```python
from build123d import *

# Parameters (mm, degrees)
SKETCH_2_R               = 2.1
SKETCH_2_R_2             = 4.1
EXTRUDE_2_DEPTH          = 3
EXTRUDE_3_DEPTH          = 15
SKETCH_4_R               = 4.1
SKETCH_4_R_2             = 2.1
EXTRUDE_4_DEPTH          = 10
EXTRUDE_START            = -13
EXTRUDE_5_DEPTH          = 13
SKETCH_7_R               = 1.3
CUT_EXTRUDE_1_DEPTH      = 13
CUT_EXTRUDE_2_DEPTH      = 174.68818701
CUT_EXTRUDE_2_DEPTH_BACK = 174.68818701
SKETCH_8_W               = 110
SKETCH_8_H               = 2.6
SKETCH_8_H_2             = 2.5
CUT_EXTRUDE_3_DEPTH      = 172.969913078
CUT_EXTRUDE_3_DEPTH_BACK = 172.969913078
EXTRUDE_6_DEPTH          = 10
SKETCH_11_R              = 2
CUT_EXTRUDE_4_DEPTH      = 10
SKETCH_13_R              = 2.05
CUT_EXTRUDE_5_DEPTH      = 10
SKETCH_14_R              = 4.1
EXTRUDE_7_DEPTH          = 3
CUT_EXTRUDE_6_DEPTH      = 3


# Read off the part's stored shape, not the designer's step: 凸台-拉伸3, 凸台-拉伸5
with BuildPart() as part:
    # 草图2 → 凸台-拉伸2 (new body)
    with BuildSketch(Plane(origin=(0, 0, 0), x_dir=(1, 0, 0), z_dir=(0, 1, 0))):
        with BuildLine():
            Line((80.099742919, 115.241133642), (-11.337123868, 9.698254241))
            ThreePointArc((-11.337123868, 9.698254241), (-10.606601718, -10.730242528), (9.821895051, -11.460764678))
            Line((9.821895051, -11.460764678), (115.364774452, 79.976102109))
            ThreePointArc((115.364774452, 79.976102109), (115.409508589, 80.014950331), (115.454150533, 80.053904459))
            Line((115.454150533, 80.053904459), (113.400395441, 82.243526883))
            ThreePointArc((113.400395441, 82.243526883), (115.041169115, 113.92185113), (83.322768112, 114.310956698))
            Line((83.322768112, 114.310956698), (81.26901302, 116.500579122))
            ThreePointArc((81.26901302, 116.500579122), (80.673552706, 115.880906565), (80.099742919, 115.241133642))
        make_face()
        with Locations(Location((98.994949366, 98.871308556, 0), (0, 0, 270))):
            Circle(SKETCH_2_R, mode=Mode.SUBTRACT)
        with Locations(Location((0, -0.12364081, 0), (0, 0, 270))):
            Circle(SKETCH_2_R_2, mode=Mode.SUBTRACT)
        with Locations(Location((70.710678119, 70.587037309, 0), (0, 0, 270))):
            Circle(SKETCH_2_R_2, mode=Mode.SUBTRACT)
    extrude(amount=EXTRUDE_2_DEPTH)

    # 凸台-拉伸3 outline → 凸台-拉伸3 (add)
    with BuildSketch(Plane(origin=(0, 3, 0), x_dir=(1, 0, 0), z_dir=(0, 1, 0))):
        with BuildLine():
            ThreePointArc((-11.337123868, 9.698254241), (-10.606601718, -10.730242528), (9.821895051, -11.460764678))
            Line((9.821895051, -11.460764678), (115.454150533, 80.053904459))
            Line((115.454150533, 80.053904459), (113.400395441, 82.243526883))
            ThreePointArc((113.400395441, 82.243526883), (113.358376595, 82.207216674), (113.316266225, 82.171012648))
            Line((113.316266225, 82.171012648), (7.857534265, -9.193324116))
            ThreePointArc((7.857534265, -9.193324116), (-8.484829636, -8.609373899), (-9.07051987, 7.732927734))
            Line((-9.07051987, 7.732927734), (81.368262538, 112.03565098))
            ThreePointArc((81.368262538, 112.03565098), (82.306692779, 113.206652712), (83.322768112, 114.310956698))
            Line((83.322768112, 114.310956698), (81.26901302, 116.500579122))
            Line((81.26901302, 116.500579122), (-11.337123868, 9.698254241))
        make_face()
    extrude(amount=EXTRUDE_3_DEPTH)

    # 草图4 → 凸台-拉伸4 (add)
    with BuildSketch(Plane(origin=(0, 3, 0), x_dir=(1, 0, 0), z_dir=(0, 1, 0))):
        with Locations(Location((98.994949366, 98.871308556, 0), (0, 0, 270))):
            Circle(SKETCH_4_R)
        with Locations(Location((98.994949366, 98.871308556, 0), (0, 0, 270))):
            Circle(SKETCH_4_R_2, mode=Mode.SUBTRACT)
    extrude(amount=EXTRUDE_4_DEPTH)

    # 凸台-拉伸5 outline → 凸台-拉伸5 (add)
    with BuildSketch(Plane(origin=(0, 13, 0), x_dir=(1, 0, 0), z_dir=(0, 1, 0)).offset(EXTRUDE_START)):
        with BuildLine():
            ThreePointArc((101.094850935, 98.891640782), (100.479873606, 100.356232796), (99.015281592, 100.971210125))
            Line((99.015281592, 100.971210125), (101.094850935, 98.891640782))
        make_face()
    extrude(amount=EXTRUDE_5_DEPTH)

    # 草图7 → 切除-拉伸1 (cut)
    with BuildSketch(Plane(origin=(99.993245858, 0, -99.993245858), x_dir=(0.7071067811865475, 0, 0.7071067811865477), z_dir=(-0.7071067811865477, 0, 0.7071067811865475))):
        with Locations((0, 5)):
            Circle(SKETCH_7_R)
    extrude(amount=-CUT_EXTRUDE_1_DEPTH, mode=Mode.SUBTRACT)

    # 草图8 → 切除-拉伸2 (cut, two sides: drawn at the far end of the back side and taken through both)
    with BuildSketch(Plane(origin=(9.883107451, 0, 11.40773322), x_dir=(0.75580694217799, 0, -0.6547945220873159), z_dir=(0.6547945220873159, 0, 0.75580694217799)).offset(-CUT_EXTRUDE_2_DEPTH_BACK)):
        with Locations((54.959520341, 10.3)):
            Rectangle(SKETCH_8_W, SKETCH_8_H)
        with Locations((54.959520341, 7.75)):
            Rectangle(SKETCH_8_W, SKETCH_8_H_2)
    extrude(amount=CUT_EXTRUDE_2_DEPTH + CUT_EXTRUDE_2_DEPTH_BACK, mode=Mode.SUBTRACT)

    # 草图9 → 切除-拉伸3 (cut, two sides: drawn at the far end of the back side and taken through both)
    with BuildSketch(Plane.XZ.offset(-CUT_EXTRUDE_3_DEPTH_BACK)):
        Polygon((83.449732713, -83.303817091), (81.326556947, -81.184353794), (67.196801633, -95.338858899), (69.319977399, -97.458322196), align=None)
        Polygon((95.456312261, -67.02984869), (81.326556947, -81.184353794), (83.449732713, -83.303817091), (97.579488027, -69.149311987), align=None)
    extrude(amount=CUT_EXTRUDE_3_DEPTH + CUT_EXTRUDE_3_DEPTH_BACK, mode=Mode.SUBTRACT)

    # 草图10 → 凸台-拉伸6 (add)
    with BuildSketch(Plane(origin=(0, 3, 0), x_dir=(1, 0, 0), z_dir=(0, 1, 0))):
        Polygon((81.326556947, 81.184353794), (70.022752696, 92.507957878), (68.182667032, 90.671089687), (79.486471284, 79.347485603), align=None)
        Polygon((92.630361199, 69.86074971), (81.326556947, 81.184353794), (79.486471284, 79.347485603), (90.790275535, 68.02388152), align=None)
        Polygon((73.986014125, 96.464289366), (72.145928462, 94.627421175), (83.449732713, 83.303817091), (94.753536964, 71.980213008), (96.593622628, 73.817081198), align=None)
    extrude(amount=EXTRUDE_6_DEPTH)

    # 草图11 → 切除-拉伸4 (cut)
    with BuildSketch(Plane(origin=(85.289818377, 0, -85.140685282), x_dir=(-0.7064877657092933, 0, -0.707725255238988), z_dir=(0.707725255238988, 0, -0.7064877657092933))):
        with Locations((-9.96499851, 8)):
            Circle(SKETCH_11_R)
        with Locations((9.96499851, 8)):
            Circle(SKETCH_11_R)
    extrude(amount=-CUT_EXTRUDE_4_DEPTH, mode=Mode.SUBTRACT)

    # 草图13 → 切除-拉伸5 (cut)
    with BuildSketch(Plane(origin=(85.289818377, 0, -85.140685282), x_dir=(-0.7064877657092933, 0, -0.707725255238988), z_dir=(0.707725255238988, 0, -0.7064877657092933))):
        with Locations((-9.96499851, 8)):
            Circle(SKETCH_13_R)
        with Locations((9.964998511, 8)):
            Circle(SKETCH_13_R)
    extrude(amount=-CUT_EXTRUDE_5_DEPTH, mode=Mode.SUBTRACT)

    # 草图14 → 凸台-拉伸7 (add)
    with BuildSketch(Plane.XZ):
        with Locations((70.710678119, -70.587037309)):
            Circle(SKETCH_14_R)
    extrude(amount=-EXTRUDE_7_DEPTH)

    # 草图15 → 切除-拉伸6 (cut)
    with BuildSketch(Plane.XZ):
        with BuildLine():
            ThreePointArc((69.902009877, -65.719825747), (67.369828397, -61.931429637), (62.901061054, -62.822500095))
            Line((62.901061054, -62.822500095), (65.802009877, -65.719825747))
            Line((65.802009877, -65.719825747), (68.702958699, -68.617151398))
            ThreePointArc((68.702958699, -68.617151398), (69.590405987, -67.287644267), (69.902009877, -65.719825747))
        make_face()
        with BuildLine():
            Line((65.802009877, -65.719825747), (62.901061054, -62.822500095))
            ThreePointArc((62.901061054, -62.822500095), (62.904684226, -68.620774569), (68.702958699, -68.617151398))
            Line((68.702958699, -68.617151398), (65.802009877, -65.719825747))
        make_face()
    extrude(amount=-CUT_EXTRUDE_6_DEPTH, mode=Mode.SUBTRACT)


solid = part.part
```
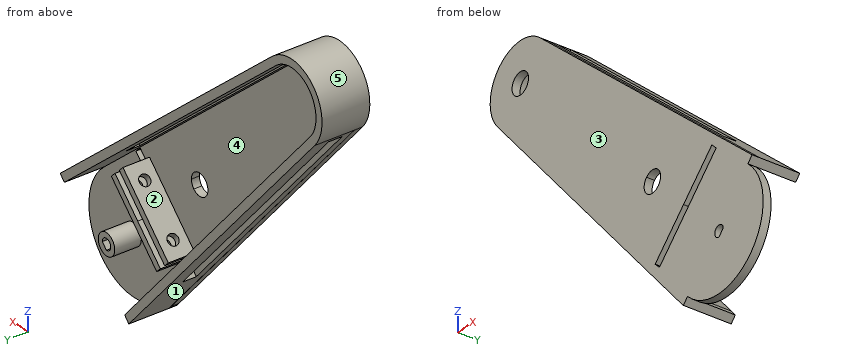
Geometry check sheet. Reference: the model listing, model coordinates, mm. Face numbers are marked on the shaded views. A direction names the side the tool comes from. Round coordinates to 2 decimals unless told otherwise and drop trailing zeros. Write each loop counter-clockwise with the first axis right and the second up, starting at its lowest first coordinate (ties: lowest second). Pieces come first, ordered by that corner, then holes. Notation, with made-up numbers: (-11, 29.5) - (11, 29.5) arc R33 cw to (11, 65.5) - close; hole circle Ø6 at (0.25, 78.25). An arc over 180 degrees is marked (long way). Write each question's results on one line, items separated by ' | '.
(1) Set-up check for the marked faces 4 and 5: record each of +Z, -Z, +X, -X, +Y, -Y from which the full face is reachable in a straight line by a thin tool's end or side.
Computed:
face 4: +Y | face 5: +Y, -Y
(2) Sectioned sample at B-B, the plane x = 51. Count the separate pieces of the cut face and the enclosed holes in it, plus the area to 3 significant figures.
Computed:
separate pieces: 3 | enclosed holes: 0 | area: 257 mm^2
(3) Depth check by flat-ended pin: pin 1 Ø10 at (x, z) = (91.5, -75.5) entering from +Y; pin 2 Ø22.5 at (x, z) = (33.5, -8) entering from -Y; pin 3 Ø6.5 at (x, z) = (0, 0.12) entering from +Y; pin 4 Ø1 at (y, z) = (3.5, -31) entering from +X. Enter the tip coordinate at first touch or a pass-through.
Computed:
pin 1: stops at y = 13 | pin 2: stops at y = 0 | pin 3: passes through | pin 4: stops at x = 59.41
(4) Draft check along Z on the marked faces 1, 2 and 3. Enter one of: pulls with the +Z half, pulls with the -Z half, needs draft (parallel to the pull), parting line crosses it, or undercut.
Computed:
face 1: pulls with the -Z half | face 2: undercut | face 3: needs draft
(5) Thickness scan on probe 1 along Z at (x, y) = (85, 12); probe 2 along X at (y, z) = (3.75, -62); probe 3 along X at (y, z) = (6, -21). Record the ranges inside material, lowest first. Write a range as from..to.
Computed:
probe 1: z = -85.43..-81.75, -77.5..-73.82, -57.64..-53.67 | probe 2: x = 34.01..37.98, 90.03..94.62 | probe 3: x = -1.54..2.43, 42.71..47.29
(6) Sectioned sample at A-A, the plane y = 15.75. Enter the section's corners in (x, z), plus the area to 3 significant figures.
Computed:
outline: (-11.34, -9.7) - (81.27, -116.5) - (83.32, -114.31) arc R22 cw to (81.37, -112.04) - (-9.07, -7.73) arc R12 cw to (7.86, 9.19) - (113.32, -82.17) arc R22 cw to (113.4, -82.24) - (115.45, -80.05) - (9.82, 11.46) arc R15 ccw to start | area: 964 mm^2
